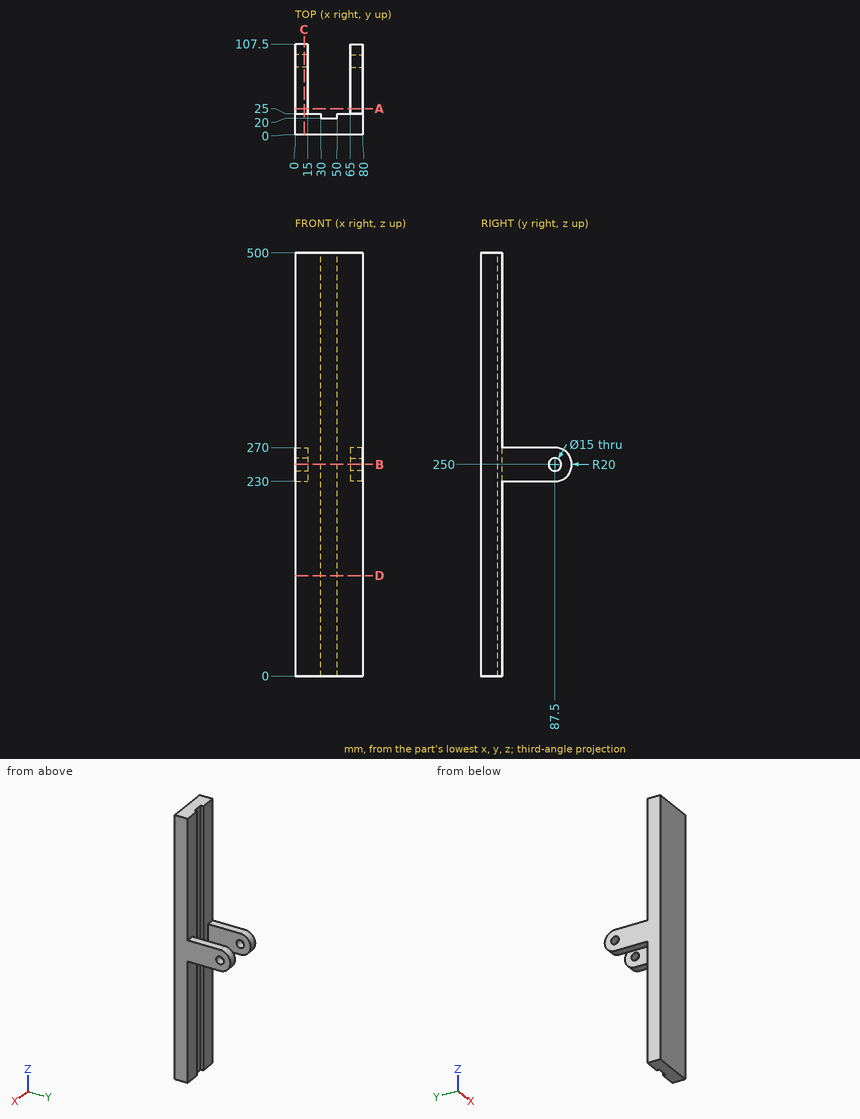
Design review of the part shown in the three views and the two pictorial views. Dimensions are in mm from the part's minimum x, y and z. Give positions to 0.01 mm unless a question says otherwise; leave off trailing zeros. Loops run counter-clockwise (first coordinate to the right, second up) from the corner with the lowest first, then second, coordinate; pieces in that order, holes last. Notation, with made-up numbers: M 25.5,8 L 45.5,8 A26 cw 45.5,36 Z; hole C 64,89.5 d10. An arc over 180 degrees is marked long. Answer as a JSON object with one key per item and string values. Group by question number.
Q1. Add section B-B on z = 250. Give the boundary of the cut face in (x, y), and give its area (4 significant figures).
Q2. Add section C-C on x = 10.5. Give the boundary of the cut face in (y, z), and give its area (3 significant figures).
Q3. For probe 1 along Y at (x, z) = (70, 250); probe 2 along Z at (x, y) = (3, 87); probe 3 along Z at (x, y) = (9.5, 29), list the stretches that pass through material, from the lowest coordinate up. Write a range as [from, to].
Q4. Add section A-A on y = 31. Give the boundary of the cut face in (x, z).
Q5. Add section D-D on z = 118.5. Give the boundary of the cut face in (x, y), and give its area (3 significant figures).
Q6. Insertion check: P1, Ø1.5, axis at x = 65.5, z = 59.5, coming from the +Y side; P2, Ø10, axis at y = 32.5, z = 73, coming from the -X side; P3, Ø7.5, axis at x = 10.5, y = 56.5, coming from the +Z side; P4, Ø16.5, axis at x = 7, y = 65.5, coming from the -Z side. Each pin has a flat end and moves straight along its axis. Give the tip position at first contact, or say it passes through.
Checked values:
{
 "1": {"outline": "M 0,0 L 80,0 L 80,80 L 65,80 L 65,25 L 50,25 L 50,20 L 30,20 L 30,25 L 15,25 L 15,80 L 0,80 Z; M 0,95 L 15,95 L 15,107.5 L 0,107.5 Z; M 65,95 L 80,95 L 80,107.5 L 65,107.5 Z", "area": "3,925 mm²"},
 "2": {"outline": "M 0,0 L 25,0 L 25,230 L 87.5,230 A20 ccw 87.5,270 L 25,270 L 25,500 L 0,500 Z; hole C 87.5,250 d15", "area": "15,500 mm²"},
 "3": {"probe 1": "[0, 80], [95, 107.5]", "probe 2": "[230, 242.52], [257.48, 270]", "probe 3": "[230, 270]"},
 "4": {"outline": "M 0,230 L 15,230 L 15,270 L 0,270 Z; M 65,230 L 80,230 L 80,270 L 65,270 Z"},
 "5": {"outline": "M 0,0 L 80,0 L 80,25 L 50,25 L 50,20 L 30,20 L 30,25 L 0,25 Z", "area": "1,900 mm²"},
 "6": {"P1": "y = 25", "P2": "through", "P3": "z = 270", "P4": "z = 230"}
}
